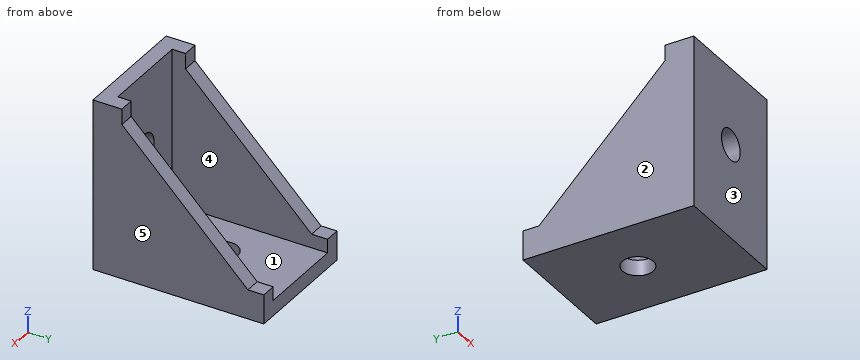
from build123d import *

# Parameters (mm, degrees)
SKETCH1_W                  = 19.812
SKETCH1_H                  = 27.94
BOSS_EXTRUDE1_DEPTH        = 27.94
SKETCH2_W                  = 14.732
SKETCH2_H                  = 25.4
CUT_EXTRUDE2_DEPTH         = 25.4
CUT_EXTRUDE3_DEPTH         = 45.201838695
CUT_EXTRUDE3_DEPTH_BACK    = 45.201838695
F_8_0_199_DIAMETER_HOLE1_D = 5.0546
F_8_0_199_DIAMETER_HOLE2_D = 5.0546


with BuildPart() as part:
    # Sketch1 → Boss-Extrude1 (new body)
    with BuildSketch(Plane.XY):
        with Locations((9.906, -13.97)):
            Rectangle(SKETCH1_W, SKETCH1_H)
    extrude(amount=BOSS_EXTRUDE1_DEPTH)

    # Sketch2 → Cut-Extrude2 (cut)
    with BuildSketch(Plane.XY.offset(27.94)):
        with Locations((9.92950186, -12.7)):
            Rectangle(SKETCH2_W, SKETCH2_H)
    extrude(amount=-CUT_EXTRUDE2_DEPTH, mode=Mode.SUBTRACT)

    # Sketch3 → Cut-Extrude3 (cut, two sides: drawn at the far end of the back side and taken through both)
    with BuildSketch(Plane(origin=(19.812, 0, 0), x_dir=(0, 0, -1), z_dir=(1, 0, 0)).offset(-CUT_EXTRUDE3_DEPTH_BACK)):
        Polygon((-27.94, 89.026253865), (-27.94, 0), (-27.94, -23.217666002), (-25.4, -23.217666002), (-4.791969325, -2.609635327), (-4.791969325, 0), (-4.791969325, 89.026253865), (-4.791969325, 267.078761596), (-27.94, 267.078761596), align=None)
    extrude(amount=CUT_EXTRUDE3_DEPTH + CUT_EXTRUDE3_DEPTH_BACK, mode=Mode.SUBTRACT)

    # #8 (0.199) Diameter Hole1 (through all)
    with Locations(Plane(origin=(0, -25.4, 0), x_dir=(1, 0, 0), z_dir=(0, 1, 0))):
        with Locations((10.016640072, -15.343780892)):
            Hole(F_8_0_199_DIAMETER_HOLE1_D / 2)

    # #8 (0.199) Diameter Hole2 (through all)
    with Locations(Plane.XY.offset(2.54)):
        with Locations((9.703159868, -12.928139324)):
            Hole(F_8_0_199_DIAMETER_HOLE2_D / 2)


solid = part.part
Work out the finished part from the listing and answer in its coordinate system (mm). Face numbers are marked on the shaded views. A direction names the side the tool comes from. Give positions to 0.01 mm unless a question says otherwise; leave off trailing zeros. Order: outer loops, then holes, each group sorted by start corner. A loop starts at its lowest first (then second) coordinate and runs counter-clockwise, first axis right, second up. Notation, with made-up numbers: M 88,45 L 114,45 A23 cw 114,77 Z; hole C 13,84.25 d9. An arc over 180 degrees is marked long. Return JSON: item names as keys, results as strings.
Q1. Find section C-C, the plane x = 5.75. Write down the section's boundary in (y, z).
Answer below:
{"outline": "M -27.94,0 L 0,0 L 0,2.54 L -25.4,2.54 L -25.4,27.94 L -27.94,27.94 Z"}
Q2. Find the intervals of material crossed by line 1 along X through (y, z) = (-6.5, 7); line 2 along Y through (x, z) = (4.25, 21.75); line 3 along Z through (x, y) = (15.5, -24), in increasing order. Write a range as [from, to].
Answer below:
{"line 1": "x = [0, 2.56], [17.3, 19.81]", "line 2": "y = [-27.94, -25.4]", "line 3": "z = [0, 2.54]"}
Q3. The mould has two halves that part along X. Classify the marked faces 3, 4 and 5: pulls with the +X half, pulls with the -X half, needs draft (parallel to the pull), parting line crosses it, or undercut.
Answer below:
{"face 3": "needs draft", "face 4": "undercut", "face 5": "pulls with the +X half"}
Q4. Find section A-A, the plane y = -12.5. Write down the section's boundary in (x, z), and give its area (3 significant figures).
Answer below:
{"outline": "M 0,0 L 7.21,0 L 7.21,2.54 L 2.56,2.54 L 2.56,14.68 L 0,14.68 Z; M 12.19,0 L 19.81,0 L 19.81,14.68 L 17.3,14.68 L 17.3,2.54 L 12.19,2.54 Z", "area": "99.4 mm^2"}
Q5. Find section B-B, the plane z = 3.5. Write down the section's boundary in (x, y), and give its area (3 significant figures).
Answer below:
{"outline": "M 0,-27.94 L 19.81,-27.94 L 19.81,0 L 17.3,0 L 17.3,-25.4 L 2.56,-25.4 L 2.56,0 L 0,0 Z", "area": "179 mm^2"}
Q6. Which of the six approach directions +Z, -Z, +X, -X, +Y, -Y give full straight-line access (tool end or side, diameter ignored) to the marked faces 1 and 2?
Answer below:
{"face 1": "+Z, +Y", "face 2": "+Z, -Z, -X, +Y, -Y"}
Q7. Find section D-D, the plane y = -23.75. Write down the section's boundary in (x, z).
Answer below:
{"outline": "M 0,0 L 19.81,0 L 19.81,27.94 L 17.3,27.94 L 17.3,2.54 L 2.56,2.54 L 2.56,27.94 L 0,27.94 Z"}
Q8. Each of these flat-tipped pins is pushed along its axis until it touches: pin 1 (0.8 mm diameter, centred on x = 19, z = 26.5, fed in from +Y); pin 2 (3 mm diameter, centred on x = 1, z = 26, fed in from +Y); pin 3 (6 mm diameter, centred on x = 10.02, z = 15.34, fed in from +Y). Where does it stop, or does it pass through?
Answer below:
{"pin 1": "stops at y = -23.22", "pin 2": "stops at y = -22.32", "pin 3": "stops at y = -25.4"}
